The listing builds one solid part. Answer for the finished solid, in the listing's coordinates (mm). Round coordinates to 2 decimals unless told otherwise and drop trailing zeros. Loops run counter-clockwise (first coordinate to the right, second up) from the corner with the lowest first, then second, coordinate; pieces in that order, holes last. Notation, with made-up numbers: M 67.5,-25 L 107.5,-25 A30 ccw 107.5,0 Z; hole C 16,-25.5 d6. An arc over 180 degrees is marked long. Put each result on its own line as item: value. Start each with the question number.
(1) Section B-B, the plane x = 0 is taken. Determine the outline of the cut face in (y, z), then the cut area to 3 significant figures.
(2) Section D-D, the plane x = 4.5 is taken. Determine the outline of the cut face in (y, z), then the cut area to 3 significant figures.
(3) A flat-ended cylindrical pin translates along its axis: P1, Ø4, axis at y = -8.5, z = 8.5, coming from the +X side. Find the tip coordinate at first contact, or state that the pin passes through.
(4) Straight lines are drawn through the part: line 1 (Z direction, x = 0, y = -5); line 2 (Z direction, x = 0, y = -5.5); line 3 (Z direction, x = 7, y = -9.25). For each, find the intervals that lie inside material, in ascending order.
(5) Section A-A, the plane z = -3.5 is taken. Determine the outline of the cut face in (x, y), then the cut area to 3 significant figures.
(6) Determine the mould class of faces 1 (the face through (-0.867, -4.93, -3.905)), 2 (the face through (9.49, -5.07, 12.27)), 3 (the face through (-12.5, -5, -10)) for opening direction Z: released by +Z, released by -Z, zero draft, split by the parting line, or undercut.
(7) Section C-C, the plane y = -6.25 is taken. Determine the outline of the cut face in (x, z), then the cut area to 3 significant figures.
```python
from build123d import *

# Parameters (mm, degrees)
F0_W     = 25
F0_H     = 40
F0_R     = 4
F1_DEPTH = 10
F3_DEPTH = 25.001
F4_R     = 10


with BuildPart() as f1:
    # F0 (on Front) → F1 (new body)
    with BuildSketch(Plane.XZ):
        with Locations((0, -4.883111)):
            Rectangle(F0_W, F0_H)
        Circle(F0_R, mode=Mode.SUBTRACT)
    extrude(amount=F1_DEPTH)

    # F2 (on face) → F3 (cut, through all)
    with BuildSketch(Plane.YZ.offset(12.5)):
        Polygon((-10, -24.883111), (0, -24.883111), (0, -22.203619), align=None)
    extrude(amount=-F3_DEPTH, mode=Mode.SUBTRACT)

    # F4
    f4_edges = [f1.edges().sort_by_distance(p)[0] for p in [
        (12.5, -5, 15.116889),
        (-12.5, -5, 15.116889),
    ]]
    fillet(f4_edges, radius=F4_R)


solid = f1.part
```
Recorded:
1. outline: M -10,-24.88 L 0,-22.2 L 0,-4 L -10,-4 Z; M -10,4 L 0,4 L 0,15.12 L -10,15.12 Z
1. area: 307 mm²
2. outline: M -10,-24.88 L 0,-22.2 L 0,14.91 L -10,14.91 Z
2. area: 385 mm²
3. P1: stops at x = 12.4
4. line 1: z = -23.54 to -4, 4 to 15.12
4. line 2: z = -23.68 to -4, 4 to 15.12
4. line 3: z = -24.68 to 14.05
5. outline: M -12.5,-10 L -1.94,-10 L -1.94,0 L -12.5,0 Z; M 1.94,-10 L 12.5,-10 L 12.5,0 L 1.94,0 Z
5. area: 211 mm²
6. face 1: undercut
6. face 2: released by +Z
6. face 3: zero draft
7. outline: M -12.5,-23.88 L 12.5,-23.88 L 12.5,5.12 A10 ccw 2.5,15.12 L -2.5,15.12 A10 ccw -12.5,5.12 Z; hole C 0,0 d8
7. area: 882 mm²
